Verification items for the finished model (mm, model axes). Face numbers are marked on the shaded views. A direction names the side the tool comes from. Round coordinates to 2 decimals unless told otherwise and drop trailing zeros. Loops run counter-clockwise (first coordinate to the right, second up) from the corner with the lowest first, then second, coordinate; pieces in that order, holes last. Notation, with made-up numbers: (43, -33.5) -> (94, -33.5) arc R20 cw to (94, -9.5) -> close; hole circle Ø3 at (88.25, 37). An arc over 180 degrees is marked (long way). Write item = value, one per line. Start each with the question number.
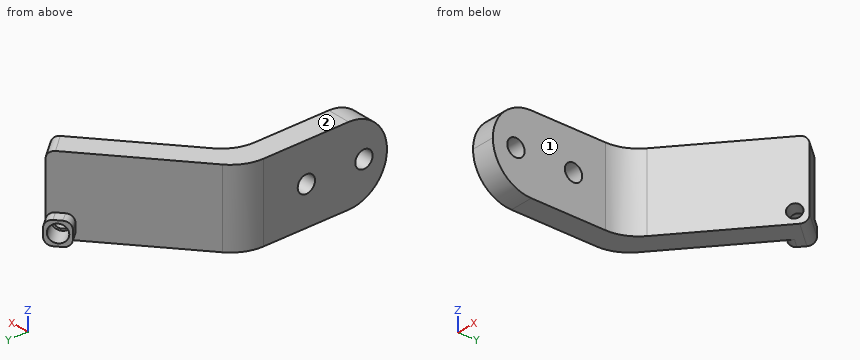
```python
from build123d import *

# Parameters (mm, degrees)
BOSS_EXTRU_1_DEPTH           = 20
ENL_V_MAT_EXTRU_1_DEPTH      = 72.5512653594726
ENL_V_MAT_EXTRU_1_DEPTH_BACK = 72.5512653594726
ESQUISSE2_R                  = 2.250000000000001
ESQUISSE2_R_2                = 2.2500000000000027
ESQUISSE3_W                  = 6
ESQUISSE3_H                  = 6
BOSS_EXTRU_2_DEPTH           = 3
ESQUISSE4_R                  = 2.249999999999996
ENL_V_MAT_EXTRU_2_DEPTH      = 5
ENL_V_MAT_EXTRU_3_DEPTH      = 71.97314065505222
ENL_V_MAT_EXTRU_3_DEPTH_BACK = 71.97314065505222
ESQUISSE5_R                  = 1.7499999999999962
CONG_1_R                     = 10
CONG_2_R                     = 2


with BuildPart() as part:
    # Esquisse1 → Boss.-Extru.1 (new body)
    with BuildSketch(Plane.XY):
        Polygon((0, 0), (0, 36.797845948930004), (30.64177772475918, 62.50935033639152), (34.498503382878404, 57.91308367767763), (5.9999999999999964, 34), (6, -9.3e-16), align=None)
    extrude(amount=BOSS_EXTRU_1_DEPTH)

    # Esquisse2 → Enlèv. mat.-Extru.1 (cut, two sides: drawn at the far end of the back side and taken through both)
    with BuildSketch(Plane(origin=(6, 6.1e-16, 0), x_dir=(0, 0, -1), z_dir=(1, 1.2e-16, 0)).offset(-ENL_V_MAT_EXTRU_1_DEPTH_BACK)):
        with Locations(Location((-10, 6.000000000000001, 0), (0, 0, 90))):
            Circle(ESQUISSE2_R)
        with Locations(Location((-10, 21, 0), (0, 0, 90))):
            Circle(ESQUISSE2_R_2)
    extrude(amount=ENL_V_MAT_EXTRU_1_DEPTH + ENL_V_MAT_EXTRU_1_DEPTH_BACK, mode=Mode.SUBTRACT)

    # Esquisse3 → Boss.-Extru.2 (add)
    with BuildSketch(Plane(origin=(-18.11940199232756, 21.59386242001515, 0), x_dir=(0.7660444431189798, 0.6427876096865373, 0), z_dir=(-0.6427876096865373, 0.7660444431189798, 0))):
        with Locations((60.65319943912616, -3)):
            Rectangle(ESQUISSE3_W, ESQUISSE3_H)
    extrude(amount=BOSS_EXTRU_2_DEPTH)

    # Esquisse4 → Enlèv. mat.-Extru.2 (cut)
    with BuildSketch(Plane(origin=(-20.047764821387148, 23.89199574937203, 0), x_dir=(0.7660444431189795, 0.6427876096865378, 0), z_dir=(-0.6427876096865378, 0.7660444431189795, 0))):
        with Locations(Location((60.653199439126226, -3, 0), (0, 0, 180))):
            Circle(ESQUISSE4_R)
    extrude(amount=-ENL_V_MAT_EXTRU_2_DEPTH, mode=Mode.SUBTRACT)

    # Esquisse5 → Enlèv. mat.-Extru.3 (cut, two sides: drawn at the far end of the back side and taken through both)
    with BuildSketch(Plane(origin=(-16.83382677295446, 20.061773533777156, 0), x_dir=(0.7660444431189792, 0.6427876096865379, 0), z_dir=(-0.6427876096865379, 0.7660444431189792, 0)).offset(-ENL_V_MAT_EXTRU_3_DEPTH_BACK)):
        with Locations(Location((60.653199439126226, -3, 0), (0, 0, 180))):
            Circle(ESQUISSE5_R)
    extrude(amount=ENL_V_MAT_EXTRU_3_DEPTH + ENL_V_MAT_EXTRU_3_DEPTH_BACK, mode=Mode.SUBTRACT)

    # Congé1
    cong_1_edges = [part.edges().sort_by_distance(p)[0] for p in [
        (5.9999999999999964, 34, 10),
        (0, 36.797845948930004, 10),
        (3, -4.7e-16, 0),
        (3, -4.7e-16, 20),
    ]]
    fillet(cong_1_edges, radius=CONG_1_R - 0.0001)  # a hair under: the kernel refuses the full size

    # Congé2
    cong_2_edges = [part.edges().sort_by_distance(p)[0] for p in [
        (32.57014055381879, 60.21121700703458, 20),
        (29.67759631022939, 63.658417001069964, 6),
        (25.081329651515517, 59.80169134295074, 0),
        (25.081329651515517, 59.80169134295074, 6.000000000000001),
        (31.60595913928899, 61.360283671713034, 0),
    ]]
    fillet(cong_2_edges, radius=CONG_2_R)


solid = part.part
```
(1) Section check A-A on y = 21. Enter the section's corners in (x, z).
(2) Section check B-B on z = 8.5. Enter the section's corners in (x, y).
(3) Scan lines: line 1 (Z direction, x = 2, y = 21); line 2 (Y direction, x = 3.35, z = 10); line 3 (X direction, y = 25, z = 17.75). Record each from-to range of solid material in increasing order. Write a range as [from, to].
(4) Access from +Z, -Z, +X, -X, +Y, -Y to the whole of each face (thin tool, end or side, straight path). Record for the marked faces 1 and 2.
(5) Section check D-D on x = 8. Enter the section's corners in (y, z).
(6) Depth check by flat-ended pin: pin 1 Ø10 at (x, y) = (9, 6.5) entering from +Z; pin 2 Ø8 at (x, z) = (11, 9.5) entering from +Y; pin 3 Ø6 at (x, z) = (30.5, 11) entering from +Y; pin 4 Ø1 at (x, z) = (11.5, 17) entering from +Y. Enter the tip coordinate at first touch or a pass-through.
(7) Section check C-C on y = 6. Enter the section's corners in (x, z), then the cut area to 3 significant figures.
Computed values:
q1.outline = (0, 0) -> (6, 0) -> (6, 7.75) -> (0, 7.75) -> close; (0, 12.25) -> (6, 12.25) -> (6, 20) -> (0, 20) -> close
q2.outline = (0, 0.11) -> (6, 0.11) -> (6, 4.32) -> (0, 4.32) -> close; (0, 7.68) -> (6, 7.68) -> (6, 19.32) -> (0, 19.32) -> close; (0, 22.68) -> (6, 22.68) -> (6, 29.34) arc R10 cw to (9.57, 37) -> (34.5, 57.91) -> (30.64, 62.51) -> (3.57, 39.8) arc R10 ccw to (0, 32.13) -> close
q3.line_1 = [0, 7.75], [12.25, 20]
q3.line_2 = [0, 3.75], [8.25, 18.75], [23.25, 39.6]
q3.line_3 = [0, 6]
q4.face_1 = +Z, -Z, +X, -Y
q4.face_2 = +Z, +X, -X, +Y, -Y
q5.outline = (35.34, 0) -> (43.51, 0) -> (43.51, 20) -> (35.34, 20) -> close
q6.pin_1 = 20
q6.pin_2 = 49.38
q6.pin_3 = 62.51
q6.pin_4 = 46.87
q7.outline = (0, 0.83) -> (6, 0.83) -> (6, 7.75) -> (0, 7.75) -> close; (0, 12.25) -> (6, 12.25) -> (6, 19.17) -> (0, 19.17) -> close
q7.area = 83.0 mm²
